```python
from build123d import *

# Parameters (mm, degrees)
SK_H0_R            = 2.75
CUT_H0_DEPTH       = 75.227920828
SK_H1_R            = 2.75
CUT_H1_DEPTH       = 75.227920828
SK_H2_R            = 2.75
CUT_H2_DEPTH       = 75.227920828
SK_H60_R           = 2.75
CUT_H60_DEPTH      = 75.227920828
SK_H180_R          = 2.75
CUT_H180_DEPTH     = 75.227920828
SK_H300_R          = 2.75
CUT_H300_DEPTH     = 75.227920828
SK_CB0_R           = 5
CUT_CB0_DEPTH      = 3.25
SK_CB1_R           = 5
CUT_CB1_DEPTH      = 3.25
SK_CB2_R           = 5
CUT_CB2_DEPTH      = 3.25
SK_GROOVE70_R      = 36.9
SK_GROOVE70_R_2    = 33.1
CUT_GROOVE70_DEPTH = 2.4
CHAMFER_C1_SIZE    = 1


with BuildPart() as part:
    # Sk_cover → Rev_cover (revolve)
    with BuildSketch(Plane(origin=(0, 0, 0), x_dir=(1, 0, 0), z_dir=(0, 1, 0)), mode=Mode.PRIVATE) as rev_cover_sk:
        with BuildLine():
            Line((10, 0), (52, 0))
            Line((52, 0), (52, -6))
            Line((52, -6), (20, -6))
            ThreePointArc((20, -6), (15.138679109, -8.383575327), (10, -10.088817))
            Line((10, -10.088817), (10, 0))
        make_face()
    revolve(rev_cover_sk.sketch.rotate(Axis((0, 0, 0), (0, 0, 1)), 180), axis=Axis((0, 0, 0), (0, 0, 1)))

    # Sk_h0 → Cut_h0 (cut, through all)
    with BuildSketch(Plane.XY):
        with Locations(Location((44, 0, 0), (0, 0, 180))):
            Circle(SK_H0_R)
    extrude(amount=CUT_H0_DEPTH, mode=Mode.SUBTRACT)

    # Sk_h1 → Cut_h1 (cut, through all)
    with BuildSketch(Plane.XY):
        with Locations(Location((-22, 38.105117767, 0), (0, 0, 180))):
            Circle(SK_H1_R)
    extrude(amount=CUT_H1_DEPTH, mode=Mode.SUBTRACT)

    # Sk_h2 → Cut_h2 (cut, through all)
    with BuildSketch(Plane.XY):
        with Locations(Location((-22, -38.105117767, 0), (0, 0, 180))):
            Circle(SK_H2_R)
    extrude(amount=CUT_H2_DEPTH, mode=Mode.SUBTRACT)

    # Sk_h60 → Cut_h60 (cut, through all)
    with BuildSketch(Plane.XY):
        with Locations(Location((22, 38.105117767, 0), (0, 0, 180))):
            Circle(SK_H60_R)
    extrude(amount=CUT_H60_DEPTH, mode=Mode.SUBTRACT)

    # Sk_h180 → Cut_h180 (cut, through all)
    with BuildSketch(Plane.XY):
        with Locations(Location((-44, 0, 0), (0, 0, 180))):
            Circle(SK_H180_R)
    extrude(amount=CUT_H180_DEPTH, mode=Mode.SUBTRACT)

    # Sk_h300 → Cut_h300 (cut, through all)
    with BuildSketch(Plane.XY):
        with Locations(Location((22, -38.105117767, 0), (0, 0, 180))):
            Circle(SK_H300_R)
    extrude(amount=CUT_H300_DEPTH, mode=Mode.SUBTRACT)

    # Sk_cb0 → Cut_cb0 (cut, symmetric)
    with BuildSketch(Plane.XY.offset(3.75)):
        with Locations((44, 0)):
            Circle(SK_CB0_R)
    extrude(amount=CUT_CB0_DEPTH, both=True, mode=Mode.SUBTRACT)

    # Sk_cb1 → Cut_cb1 (cut, symmetric)
    with BuildSketch(Plane.XY.offset(3.75)):
        with Locations((-22, 38.105117767)):
            Circle(SK_CB1_R)
    extrude(amount=CUT_CB1_DEPTH, both=True, mode=Mode.SUBTRACT)

    # Sk_cb2 → Cut_cb2 (cut, symmetric)
    with BuildSketch(Plane.XY.offset(3.75)):
        with Locations((-22, -38.105117767)):
            Circle(SK_CB2_R)
    extrude(amount=CUT_CB2_DEPTH, both=True, mode=Mode.SUBTRACT)

    # Sk_groove70 → Cut_groove70 (cut)
    with BuildSketch(Plane.XY):
        Circle(SK_GROOVE70_R)
        Circle(SK_GROOVE70_R_2, mode=Mode.SUBTRACT)
    extrude(amount=CUT_GROOVE70_DEPTH, mode=Mode.SUBTRACT)

    # Chamfer_C1
    chamfer_c1_edges = [part.edges().sort_by_distance(p)[0] for p in [
        (52, 0, 6),
        (52, 0, 0),
    ]]
    chamfer(chamfer_c1_edges, length=CHAMFER_C1_SIZE)


solid = part.part
```
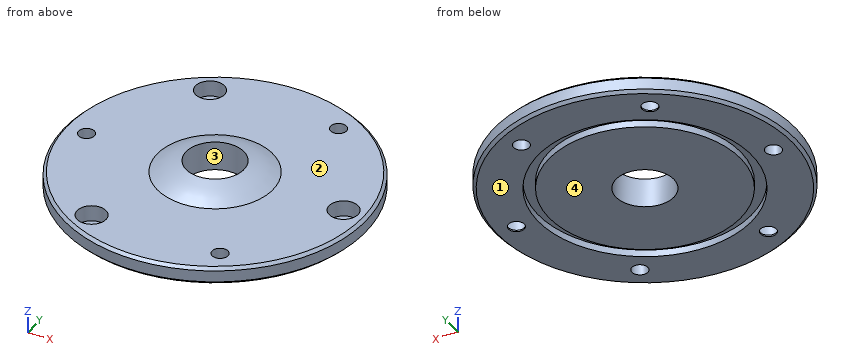
Part model, mm, in its own coordinate system. Face numbers are marked on the shaded views. A direction names the side the tool comes from. Round coordinates to 2 decimals unless told otherwise and drop trailing zeros.
1. Two-plate mould, pull along X, no slides. Class the marked faces 3 and 4: pulls with the +X half, pulls with the -X half, needs draft (parallel to the pull), parting line crosses it, or undercut.
Solutions:
face 3: undercut
face 4: needs draft
2. Drill centre lines: line 1 along X through (y, z) = (-40.5, 1); line 2 along Y through (x, z) = (22, 4.4); line 3 along X through (y, z) = (-19, 1.25). Where is each one in solid material? Low to high.
Solutions:
line 1: x = -32.62 to -26.39, -17.61 to 20.65, 23.35 to 32.62
line 2: y = -47.12 to -40.86, -35.36 to 35.36, 40.86 to 47.12
line 3: x = -48.4 to -31.63, -27.1 to 27.1, 31.63 to 48.4
3. Slice it at A-A (y = 0). Count the separate pieces of the cut face and the enclosed holes in it, and give its area (3 significant figures).
Solutions:
separate pieces: 4
enclosed holes: 0
area: 439 mm2
4. 3-axis set-ups, long thin cutter, end or side, ignore diameter. For the marked faces 1 and 2: which of +Z, -Z, +X, -X, +Y, -Y reach the whole face in a straight line?
Solutions:
face 1: -Z, +X, -X, +Y, -Y
face 2: +Z
5. Flat gauge pins, fed straight in: pin 1 (13 mm diameter, centred on x = 44, y = 0, fed in from +Z); pin 2 (3.5 mm diameter, centred on x = 44, y = 0, fed in from +Z); pin 3 (3 mm diameter, centred on x = -30.5, z = 4.5, fed in from -Y); pin 4 (9 mm diameter, centred on x = -22, y = 38.11, fed in from +Z). Where does each tip first touch, or does it go through?
Solutions:
pin 1: stops at z = 6
pin 2: passes through
pin 3: stops at y = -43.16
pin 4: stops at z = 0.5
